```python
from build123d import *

# Parameters (mm, degrees)
SKETCH1_W           = 88.9
SKETCH1_H           = 83.82
BOSS_EXTRUDE1_DEPTH = 15.875
SKETCH2_R           = 3.2639
SKETCH2_R_2         = 15.875
CUT_EXTRUDE1_DEPTH  = 16.875
SKETCH3_R           = 25.4
CUT_EXTRUDE2_DEPTH  = 12.7


with BuildPart() as part:
    # Sketch1 → Boss-Extrude1 (new body)
    with BuildSketch(Plane.XY):
        Rectangle(SKETCH1_W, SKETCH1_H)
    extrude(amount=BOSS_EXTRUDE1_DEPTH)

    # Sketch2 → Cut-Extrude1 (cut, through all)
    with BuildSketch(Plane.XY.offset(15.875)):
        with Locations((-31.75, 31.75)):
            Circle(SKETCH2_R)
        with Locations((31.75, 31.75)):
            Circle(SKETCH2_R)
        with Locations((31.75, -31.75)):
            Circle(SKETCH2_R)
        with Locations((-31.75, -31.75)):
            Circle(SKETCH2_R)
        Circle(SKETCH2_R_2)
    extrude(amount=-CUT_EXTRUDE1_DEPTH, mode=Mode.SUBTRACT)

    # Sketch3 → Cut-Extrude2 (cut)
    with BuildSketch(Plane.XY.offset(15.875)):
        Circle(SKETCH3_R)
    extrude(amount=-CUT_EXTRUDE2_DEPTH, mode=Mode.SUBTRACT)


solid = part.part
```
The listing builds one solid part. Answer for the finished solid, in the listing's coordinates (mm). A direction names the side the tool comes from. Coordinates: 2 decimals unless noted, no trailing zeros. Loops run counter-clockwise (first coordinate to the right, second up) from the corner with the lowest first, then second, coordinate; pieces in that order, holes last. Notation, with made-up numbers: M -32,44 L -21,44 A26 cw -21,76 Z; hole C 7,-4 d3. An arc over 180 degrees is marked long. Answer as CSV lines item,"result". Start each with the question number.
(1) The part is cut by section D-D (x = -1). Give the vertices of the cut face in (y, z) (3 decimals), and give its area (3 significant figures).
(2) Given pin 1 (1.5 mm diameter, centred on x = 31, y = -29, fed in from +Z) (3 decimals); pin 2 (5 mm diameter, centred on x = -31.75, y = -31.75, fed in from -Z), each flat-ended and moving along its own axis, determine where each tip first touches the part or whether it passes through.
(3) The part is cut by section B-B (x = 31.75). Give the vertices of the cut face in (y, z) (3 decimals).
(4) The part is cut by section C-C (z = 5.75). Give the vertices of the cut face in (x, y), and give its area (3 significant figures).
(5) The part is cut by section A-A (y = -31.75). Give the vertices of the cut face in (x, z) (3 decimals), and give its area (3 significant figures).
(6) For faces 1 (the flat face through (11, 12, 3.175)), 2 (the cylindrical face through (29.16, 29.764, 8.049)), determine the directions among +Z, -Z, +X, -X, +Y, -Y from which every point of the face is accessible in a straight line to the end or side of a thin tool.
(7) Find the intervals of material crossed by L1, parallel to Y at x = -31.75, z = 9.5; L2, parallel to X at y = 32, z = 7; L3, parallel to X at y = -30.5, z = 1.75, in increasing order. Write a range as [from, to].
(8) The mould has two halves that part along X. Classify faces 3 (the cylindrical face through (-32.175, -28.514, 8.049)), 4 (the flat face through (-44.45, -1, 8)), 5 (the flat face through (44.45, -1, 8)): pulls with the +X half, pulls with the -X half, needs draft (parallel to the pull), parting line crosses it, or undercut.
Determined:
1,outline,"M -41.91,0 L -15.843,0 L -15.843,3.175 L -25.38,3.175 L -25.38,15.875 L -41.91,15.875 Z; M 15.843,0 L 41.91,0 L 41.91,15.875 L 25.38,15.875 L 25.38,3.175 L 15.843,3.175 Z"
1,area,"585 mm2"
2,pin 1,"z = 15.875"
2,pin 2,"through"
3,outline,"M -41.91,0 L -35.014,0 L -35.014,15.875 L -41.91,15.875 Z; M -28.486,0 L 28.486,0 L 28.486,15.875 L -28.486,15.875 Z; M 35.014,0 L 41.91,0 L 41.91,15.875 L 35.014,15.875 Z"
4,outline,"M -44.45,-41.91 L 44.45,-41.91 L 44.45,41.91 L -44.45,41.91 Z; hole C -31.75,-31.75 d6.53; hole C -31.75,31.75 d6.53; hole C 0,0 d50.8; hole C 31.75,-31.75 d6.53; hole C 31.75,31.75 d6.53"
4,area,"5,290 mm2"
5,outline,"M -44.45,0 L -35.014,0 L -35.014,15.875 L -44.45,15.875 Z; M -28.486,0 L 28.486,0 L 28.486,15.875 L -28.486,15.875 Z; M 35.014,0 L 44.45,0 L 44.45,15.875 L 35.014,15.875 Z"
5,area,"1,200 mm2"
6,face 1,"+Z"
6,face 2,"+Z, -Z"
7,L1,"[-41.91, -35.01], [-28.49, 28.49], [35.01, 41.91]"
7,L2,"[-44.45, -35], [-28.5, 28.5], [35, 44.45]"
7,L3,"[-44.45, -34.77], [-28.73, 28.73], [34.77, 44.45]"
8,face 3,"undercut"
8,face 4,"pulls with the -X half"
8,face 5,"pulls with the +X half"
